Model file for the job. Use its own axes, mm. A direction names the side the tool comes from. Give positions to 0.01 mm unless a question says otherwise; leave off trailing zeros. Loops run counter-clockwise (first coordinate to the right, second up) from the corner with the lowest first, then second, coordinate; pieces in that order, holes last. Notation, with made-up numbers: (-26, 89) - (31, 89) arc R25 ccw to (31, 110) - close; hole circle Ø10 at (64.5, 8). An arc over 180 degrees is marked (long way). Use a Markdown table: item, result.
from build123d import *

# Parameters (mm, degrees)
F0_W     = 83
F0_H     = 26
F0_W_2   = 67
F0_H_2   = 16
F1_DEPTH = 2
F2_W     = 77
F2_H     = 20
F2_W_2   = 67
F2_H_2   = 16
F3_DEPTH = 1.5
F4_R     = 1
F5_DEPTH = 25
F6_R     = 1
F7_DEPTH = 2


with BuildPart() as f1:
    # F0 (on Top) → F1 (new body)
    with BuildSketch(Plane.XY):
        Rectangle(F0_W, F0_H)
        Rectangle(F0_W_2, F0_H_2, mode=Mode.SUBTRACT)
    extrude(amount=F1_DEPTH)

    # F2 (on face) → F3 (join)
    with BuildSketch(Plane.XY.offset(2)):
        Rectangle(F2_W, F2_H)
        Rectangle(F2_W_2, F2_H_2, mode=Mode.SUBTRACT)
    extrude(amount=F3_DEPTH)

    # F4 (on face) → F5 (cut)
    with BuildSketch(Plane(origin=(0, 0, 0), x_dir=(1, 0, 0), z_dir=(0, 0, -1))):
        with Locations((-36, 0)):
            Circle(F4_R)
        with Locations((36, 0)):
            Circle(F4_R)
    extrude(amount=-F5_DEPTH, mode=Mode.SUBTRACT)

    # F6 (on face) → F7 (cut)
    with BuildSketch(Plane(origin=(0, 0, 0), x_dir=(1, 0, 0), z_dir=(0, 0, -1))):
        with Locations((-36, 0)):
            Circle(F6_R)
        with Locations((36, 0)):
            Circle(F6_R)
        with BuildLine():
            Line((-33.5, -1.658312), (-33.5, 1.658312))
            ThreePointArc((-33.5, 1.658312), (-39, 0), (-33.5, -1.658312))
        make_face()
        with Locations((-36, 0)):
            Circle(F6_R, mode=Mode.SUBTRACT)
        with BuildLine():
            Line((33.5, -1.658312), (33.5, 1.658312))
            ThreePointArc((33.5, 1.658312), (33, 0), (33.5, -1.658312))
        make_face()
        with BuildLine():
            ThreePointArc((39, 0), (36.866025, 2.872281), (33.5, 1.658312))
            Line((33.5, 1.658312), (33.5, -1.658312))
            ThreePointArc((33.5, -1.658312), (36.866025, -2.872281), (39, 0))
        make_face()
        with Locations((36, 0)):
            Circle(F6_R, mode=Mode.SUBTRACT)
    extrude(amount=-F7_DEPTH, mode=Mode.SUBTRACT)


solid = f1.part
(1) Slice it at B-B, the plane y = -4.5. Write the cut outline in (x, z).
Computed:
| item | result |
|---|---|
| outline | (-41.5, 0) - (-33.5, 0) - (-33.5, 3.5) - (-38.5, 3.5) - (-38.5, 2) - (-41.5, 2) - close; (33.5, 0) - (41.5, 0) - (41.5, 2) - (38.5, 2) - (38.5, 3.5) - (33.5, 3.5) - close |
(2) Slice it at A-A, the plane x = 36. Write the cut outline in (y, z), plus the area to 3 significant figures.
Computed:
| item | result |
|---|---|
| outline | (-13, 0) - (-3, 0) - (-3, 2) - (-1, 2) - (-1, 3.5) - (-10, 3.5) - (-10, 2) - (-13, 2) - close; (1, 2) - (3, 2) - (3, 0) - (13, 0) - (13, 2) - (10, 2) - (10, 3.5) - (1, 3.5) - close |
| area | 67.0 mm² |
(3) Slice it at C-C, the plane z = 2.55. Write the cut outline in (x, y).
Computed:
| item | result |
|---|---|
| outline | (-38.5, -10) - (38.5, -10) - (38.5, 10) - (-38.5, 10) - close; hole circle Ø2 at (-36, 0); hole (-33.5, -8) - (33.5, -8) - (33.5, 8) - (-33.5, 8) - close; hole circle Ø2 at (36, 0) |
(4) Drill centre lines: probe 1 along X at (y, z) = (0, 2.6); probe 2 along Y at (x, z) = (36, 0.4); probe 3 along X at (y, z) = (-4.75, 2.9). Where is each one in solid material? Low to high. Write a range as [from, to].
Computed:
| item | result |
|---|---|
| probe 1 | [-38.5, -37], [-35, -33.5], [33.5, 35], [37, 38.5] |
| probe 2 | [-13, -3], [3, 13] |
| probe 3 | [-38.5, -33.5], [33.5, 38.5] |
(5) Slice it at D-D, the plane y = -9.25. Write the cut outline in (x, z).
Computed:
| item | result |
|---|---|
| outline | (-41.5, 0) - (41.5, 0) - (41.5, 2) - (38.5, 2) - (38.5, 3.5) - (-38.5, 3.5) - (-38.5, 2) - (-41.5, 2) - close |
(6) Pin check, flat tips, straight feed: P1, Ø1.2, axis at x = -18, z = 3, coming from the +Y side; P2, Ø4, axis at x = -36, y = 0.5, coming from the -Z side. Stop position of each tip, or through.
Computed:
| item | result |
|---|---|
| P1 | y = 10 |
| P2 | z = 2 |
(7) Mould opens along Y. For faces 5 (the flat face through (-41.5, 0, 1)), 6 (the flat face through (-1, -10, 3)), 7 (the flat face through (34.85, -0.04, 2)) say: pulls with the +Y half, pulls with the -Y half, needs draft (parallel to the pull), parting line crosses it, or undercut.
Computed:
| item | result |
|---|---|
| face 5 | needs draft |
| face 6 | pulls with the -Y half |
| face 7 | undercut |
(8) 3-axis set-ups, long thin cutter, end or side, ignore diameter. For faces 1 (the flat face through (0, -8, 2)), 2 (the flat face through (-1, 10, 3)), 3 (the cylindrical face through (-39, 0, 1)), 4 (the flat face through (38.5, 0, 3)): which of +Z, -Z, +X, -X, +Y, -Y reach the whole face in a straight line?
Computed:
| item | result |
|---|---|
| face 1 | +Z, -Z |
| face 2 | +Z, +X, -X, +Y |
| face 3 | -Z |
| face 4 | +Z, +X, +Y, -Y |
